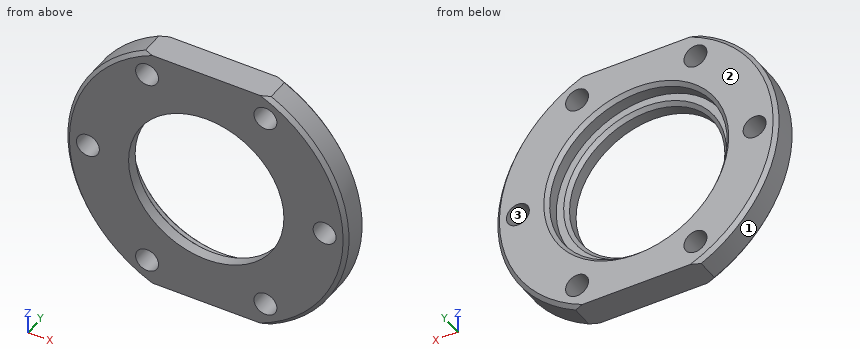
from build123d import *

# Parameters (mm, degrees)
SKETCH1_R           = 10.5
SKETCH1_R_2         = 1.55
BOSS_EXTRUDE1_DEPTH = 4
SKETCH2_R           = 12
CUT_EXTRUDE1_DEPTH  = 2
CHAMFER1_SIZE       = 0.5


with BuildPart() as part:
    # Sketch1 → Boss-Extrude1 (new body)
    with BuildSketch(Plane(origin=(0, 0, 0), x_dir=(1, 0, 0), z_dir=(0, 1, 0))):
        with BuildLine():
            Line((-8.485281374, 17), (8.485281374, 17))
            ThreePointArc((8.485281374, 17), (19, 0), (8.485281374, -17))
            Line((8.485281374, -17), (-8.485281374, -17))
            ThreePointArc((-8.485281374, -17), (-19, 0), (-8.485281374, 17))
        make_face()
        with Locations(Location((0, 0, 0), (0, 0, 270))):
            Circle(SKETCH1_R, mode=Mode.SUBTRACT)
        with Locations(Location((-16, 0, 0), (0, 0, 270))):
            Circle(SKETCH1_R_2, mode=Mode.SUBTRACT)
        with Locations(Location((-8, 13.856406461, 0), (0, 0, 270))):
            Circle(SKETCH1_R_2, mode=Mode.SUBTRACT)
        with Locations(Location((8, 13.856406461, 0), (0, 0, 270))):
            Circle(SKETCH1_R_2, mode=Mode.SUBTRACT)
        with Locations(Location((16, 0, 0), (0, 0, 270))):
            Circle(SKETCH1_R_2, mode=Mode.SUBTRACT)
        with Locations(Location((8, -13.856406461, 0), (0, 0, 270))):
            Circle(SKETCH1_R_2, mode=Mode.SUBTRACT)
        with Locations(Location((-8, -13.856406461, 0), (0, 0, 270))):
            Circle(SKETCH1_R_2, mode=Mode.SUBTRACT)
    extrude(amount=BOSS_EXTRUDE1_DEPTH)

    # Sketch2 → Cut-Extrude1 (cut)
    with BuildSketch(Plane(origin=(0, 4, 0), x_dir=(1, 0, 0), z_dir=(0, 1, 0))):
        with Locations(Location((0, 0, 0), (0, 0, 270))):
            Circle(SKETCH2_R)
    extrude(amount=-CUT_EXTRUDE1_DEPTH, mode=Mode.SUBTRACT)

    # Chamfer1
    chamfer1_edges = [part.edges().sort_by_distance(p)[0] for p in [
        (-19, 4, 0),
        (0, 2, -10.5),
        (0, 4, -12),
        (19, 4, 0),
        (-19, 0, 0),
        (19, 0, 0),
    ]]
    chamfer(chamfer1_edges, length=CHAMFER1_SIZE)


solid = part.part
The model under review builds one solid part; all positions refer to its coordinate system, in mm. Face numbers are marked on the shaded views. Round coordinates to 2 decimals unless told otherwise and drop trailing zeros. Loops run counter-clockwise (first coordinate to the right, second up) from the corner with the lowest first, then second, coordinate; pieces in that order, holes last. Notation, with made-up numbers: M 31.25,51.25 L 69.25,51.25 A33 cw 69.25,83.25 Z; hole C 59.25,33 d2. An arc over 180 degrees is marked long. Answer as CSV lines item,"result". Start each with the question number.
Item 1: Consider section C-C (z = -14). State how many separate pieces and enclosed holes the cut face has, then the cut area to 3 significant figures.
Item 2: Consider section B-B (y = 2.8). Write out the cut boundary in (x, z).
Item 3: Mouldability with a two-part tool opening along Z and no side actions: class the marked faces 1, 2 and 3 as released by +Z, released by -Z, zero draft, split by the parting line, or undercut.
Item 4: Insertion check: P1, Ø3, axis at x = -8, z = -13.86, coming from the -Y side. The pin has a flat end and moves straight along its axis. Give the tip position at first contact, or say it passes through.
Item 5: Consider section A-A (x = 0). Write out the cut boundary in (y, z).
Item 6: Wall thickness on line 1 (Z direction, x = 7, y = 3.55); line 2 (X direction, y = 2.55, z = -2.5); line 3 (X direction, y = 2.15, z = -9): over which ranges is each line inside the solid? List them lowest first. Write a range as [from, to].
Item 7: Consider section D-D (y = 1). Write out the cut boundary in (x, z).
Answer:
1,separate pieces,"3"
1,enclosed holes,"0"
1,area,"77.3 mm^2"
2,outline,"M -8.49,-17 L 8.49,-17 A19 ccw 8.49,17 L -8.49,17 A19 ccw Z; hole C -16,0 d3.1; hole C 0,0 d24; hole C -8,-13.86 d3.1; hole C -8,13.86 d3.1; hole C 8,-13.86 d3.1; hole C 8,13.86 d3.1; hole C 16,0 d3.1"
3,face 1,"split by the parting line"
3,face 2,"zero draft"
3,face 3,"undercut"
4,P1,"passes through"
5,outline,"M 0,-17 L 4,-17 L 4,-12.5 L 3.5,-12 L 2,-12 L 2,-11 L 1.5,-10.5 L 0,-10.5 Z; M 0,10.5 L 1.5,10.5 L 2,11 L 2,12 L 3.5,12 L 4,12.5 L 4,17 L 0,17 Z"
6,line 1,"z = [-17, -15.04], [-12.67, -9.81], [9.81, 12.67], [15.04, 17]"
6,line 2,"x = [-18.83, -11.74], [11.74, 18.83]"
6,line 3,"x = [-16.73, -7.94], [7.94, 16.73]"
7,outline,"M -8.49,-17 L 8.49,-17 A19 ccw 8.49,17 L -8.49,17 A19 ccw Z; hole C -16,0 d3.1; hole C 0,0 d21; hole C -8,-13.86 d3.1; hole C -8,13.86 d3.1; hole C 8,-13.86 d3.1; hole C 8,13.86 d3.1; hole C 16,0 d3.1"
